Answer from the drawing. Dimensions are ordinates in mm from the lowest x, y and z of the part. A direction names the side the tool comes from. Give positions to 0.01 mm unless a question says otherwise; leave off trailing zeros. Order: outer loops, then holes, each group sorted by start corner. A loop starts at its lowest first (then second) coordinate and runs counter-clockwise, first axis right, second up. Notation, with made-up numbers: (42.25, -13) - (64.25, -13) arc R16 cw to (64.25, -1) - close; hole circle Ø4 at (-2.5, 30). An arc over 180 degrees is marked (long way). Answer in a Markdown table with one row per item.
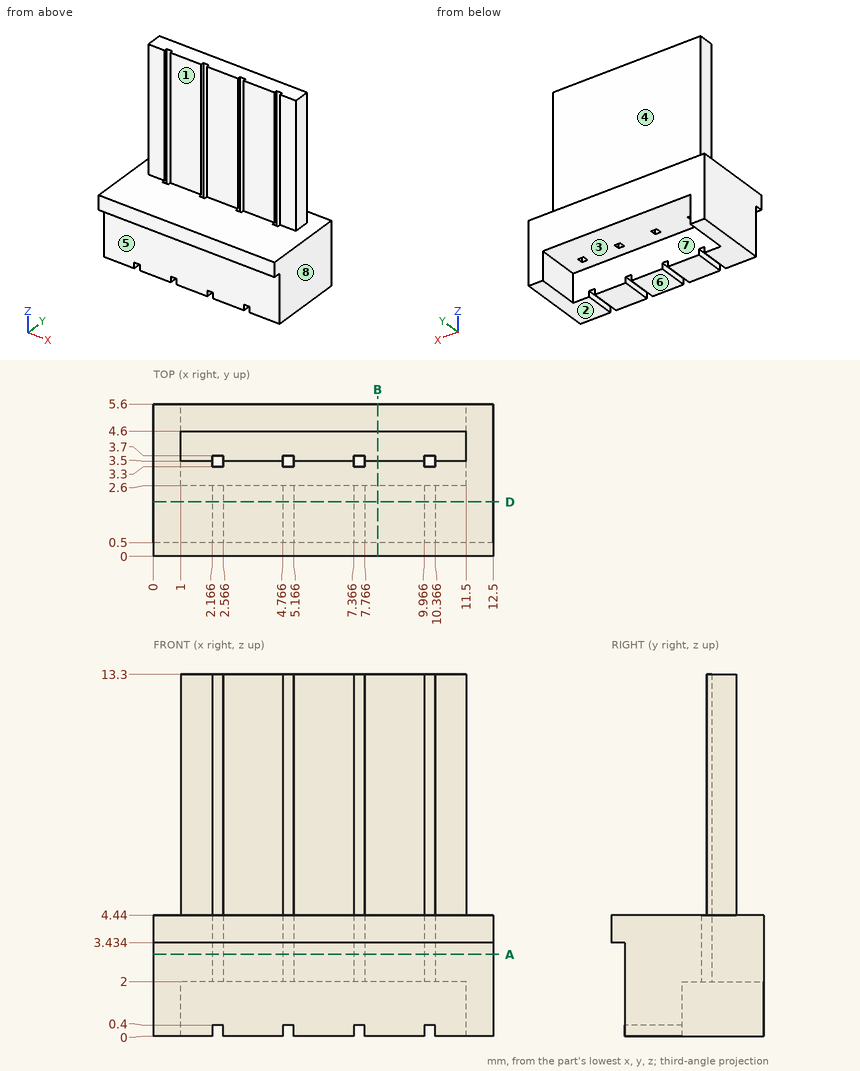
Item 1: Find section A-A on z = 3. Write down the section's boundary in (x, y) (1 decimal), then the cut area to 3 significant figures.
Answer block:
| item | result |
|---|---|
| outline | (0, 0.5) - (12.5, 0.5) - (12.5, 5.6) - (0, 5.6) - close; hole (2.2, 3.3) - (2.6, 3.3) - (2.6, 3.7) - (2.2, 3.7) - close; hole (4.8, 3.3) - (5.2, 3.3) - (5.2, 3.7) - (4.8, 3.7) - close; hole (7.4, 3.3) - (7.8, 3.3) - (7.8, 3.7) - (7.4, 3.7) - close; hole (10, 3.3) - (10.4, 3.3) - (10.4, 3.7) - (10, 3.7) - close |
| area | 63.1 mm² |
Item 2: Find section D-D on y = 2. Write down the section's boundary in (x, z) (1 decimal).
Answer block:
| item | result |
|---|---|
| outline | (0, 0) - (2.2, 0) - (2.2, 0.4) - (2.6, 0.4) - (2.6, 0) - (4.8, 0) - (4.8, 0.4) - (5.2, 0.4) - (5.2, 0) - (7.4, 0) - (7.4, 0.4) - (7.8, 0.4) - (7.8, 0) - (10, 0) - (10, 0.4) - (10.4, 0.4) - (10.4, 0) - (12.5, 0) - (12.5, 4.4) - (0, 4.4) - close |
Item 3: Which of the six approach directions +Z, -Z, +X, -X, +Y, -Y give full straight-line access (tool end or side, diameter ignored) to the marked faces 1, 2, 3, 4 and 5?
Answer block:
| item | result |
|---|---|
| face 1 | +Z, +X, -X, -Y |
| face 2 | -Z, +X, -X, +Y, -Y |
| face 3 | -Z, +Y |
| face 4 | +Z, +X, -X, +Y |
| face 5 | -Z, +X, -X, -Y |
Item 4: Find section B-B on x = 8.25. Write down the section's boundary in (y, z) (1 decimal).
Answer block:
| item | result |
|---|---|
| outline | (0, 3.4) - (0.5, 3.4) - (0.5, 0) - (2.6, 0) - (2.6, 2) - (5.6, 2) - (5.6, 4.4) - (4.6, 4.4) - (4.6, 13.3) - (3.5, 13.3) - (3.5, 4.4) - (0, 4.4) - close |
Item 5: Determine the mould class of the marked faces 6, 7 and 8 for opening direction X: pulls with the +X half, pulls with the -X half, needs draft (parallel to the pull), parting line crosses it, or undercut.
Answer block:
| item | result |
|---|---|
| face 6 | needs draft |
| face 7 | undercut |
| face 8 | pulls with the +X half |
Item 6: Each of these flat-tipped pins is pushed along its axis until it touches: P1, Ø0.7, axis at x = 3.5, z = 9, coming from the -Y side; P2, Ø6, axis at x = 7.5, z = 2.5, coming from the -Y side; P3, Ø0.9, axis at x = 4, y = 4, coming from the -Z side; P4, Ø3, axis at x = 2.5, y = 1, coming from the +Z side. Where does it stop, or does it pass through?
Answer block:
| item | result |
|---|---|
| P1 | y = 3.5 |
| P2 | y = 0 |
| P3 | z = 2 |
| P4 | z = 4.44 |
Item 7: Consider line 1 (X direction, y = 3.65, z = 6.75) (1 decimal); line 2 (Y direction, x = 3.25, z = 3); line 3 (Y direction, x = 4.5, z = 7). Determine where each line is inside the solid, lowest interval first.
Answer block:
| item | result |
|---|---|
| line 1 | 1 to 2.2, 2.6 to 4.8, 5.2 to 7.4, 7.8 to 10, 10.4 to 11.5 |
| line 2 | 0.5 to 5.6 |
| line 3 | 3.5 to 4.6 |
